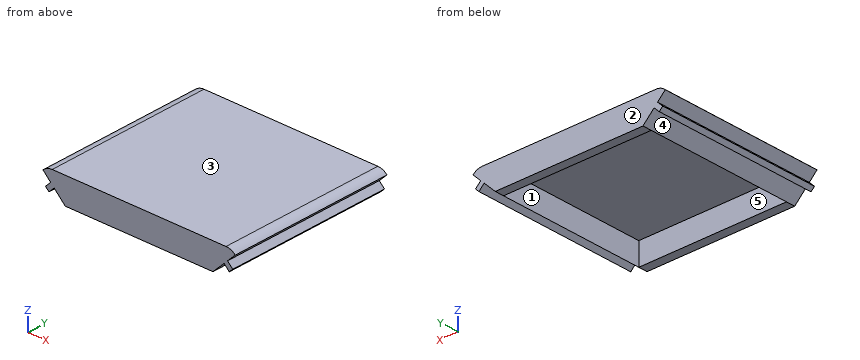
```python
from build123d import *

# Parameters (mm, degrees)
SKETCH_1_W          = 81.9
SKETCH_1_H          = 67.9
EXTRUDE_1_DEPTH     = 10.7
SKETCH_2_W          = 60.5
SKETCH_2_H          = 60.5
CUT_EXTRUDE_1_DEPTH = 9.2
CUT_EXTRUDE_2_REACH = 82.011
CUT_EXTRUDE_4_REACH = 91.242
EXTRUDE_2_DEPTH     = 67.9


with BuildPart() as part:
    # Эскиз1 → Бобышка-Вытянуть1 (new body)
    with BuildSketch(Plane.XY):
        Rectangle(SKETCH_1_W, SKETCH_1_H)
    extrude(amount=-EXTRUDE_1_DEPTH)

    # Эскиз2 → Вырез-Вытянуть1 (cut)
    with BuildSketch(Plane(origin=(0, 0, -10.7), x_dir=(-1, 0, 0), z_dir=(0, 0, -1))):
        Rectangle(SKETCH_2_W, SKETCH_2_H)
    extrude(amount=-CUT_EXTRUDE_1_DEPTH, mode=Mode.SUBTRACT)

    # Эскиз3 → Вырез-Вытянуть2 (cut, up to next)
    with BuildSketch(Plane(origin=(0, 33.95, 0), x_dir=(1, 0, 0), z_dir=(0, 1, 0)), mode=Mode.PRIVATE) as cut_extrude_2_sk1:
        Polygon((-40.95, 0), (-30.25, 10.7), (-40.95, 10.7), align=None)
    cut_extrude_2_tool1 = extrude(cut_extrude_2_sk1.sketch, amount=-CUT_EXTRUDE_2_REACH, mode=Mode.PRIVATE) & part.part
    # Эскиз3 → Вырез-Вытянуть2 (cut, up to next)
    with BuildSketch(Plane(origin=(0, 33.95, 0), x_dir=(1, 0, 0), z_dir=(0, 1, 0)), mode=Mode.PRIVATE) as cut_extrude_2_sk2:
        Polygon((40.95, 10.7), (40.95, 0), (30.25, 10.7), align=None)
    cut_extrude_2_tool2 = extrude(cut_extrude_2_sk2.sketch, amount=-CUT_EXTRUDE_2_REACH, mode=Mode.PRIVATE) & part.part
    add(cut_extrude_2_tool1.solids().sort_by_distance((-37.383333, 33.95, -7.133333))[0], mode=Mode.SUBTRACT)
    add(cut_extrude_2_tool2.solids().sort_by_distance((37.383333, 33.95, -7.133333))[0], mode=Mode.SUBTRACT)

    # Эскиз4 → Вырез-Вытянуть4 (cut, up to next)
    with BuildSketch(Plane(origin=(0, -33.95, -40.95), x_dir=(1, 0, 0), z_dir=(0, 1, 0)), mode=Mode.PRIVATE) as cut_extrude_4_sk1:
        with BuildLine():
            Line((39.383021279, -39.383021279), (40.95, -40.95))
            Line((40.95, -40.95), (35.6, -40.95))
            ThreePointArc((35.6, -40.95), (37.647356363, -40.542755499), (39.383021279, -39.383021279))
        make_face()
    cut_extrude_4_tool1 = extrude(cut_extrude_4_sk1.sketch, amount=CUT_EXTRUDE_4_REACH, mode=Mode.PRIVATE) & part.part
    # Эскиз4 → Вырез-Вытянуть4 (cut, up to next)
    with BuildSketch(Plane(origin=(0, -33.95, -40.95), x_dir=(1, 0, 0), z_dir=(0, 1, 0)), mode=Mode.PRIVATE) as cut_extrude_4_sk2:
        with BuildLine():
            Line((-40.95, -40.95), (-35.6, -40.95))
            ThreePointArc((-35.6, -40.95), (-37.647356363, -40.542755499), (-39.383021279, -39.383021279))
            Line((-39.383021279, -39.383021279), (-40.95, -40.95))
        make_face()
    cut_extrude_4_tool2 = extrude(cut_extrude_4_sk2.sketch, amount=CUT_EXTRUDE_4_REACH, mode=Mode.PRIVATE) & part.part
    add(cut_extrude_4_tool1.solids().sort_by_distance((39.042099, -33.95, -0.482136))[0], mode=Mode.SUBTRACT)
    add(cut_extrude_4_tool2.solids().sort_by_distance((-39.042099, -33.95, -0.482136))[0], mode=Mode.SUBTRACT)

    # Эскиз7 → Бобышка-Вытянуть2 (add)
    with BuildSketch(Plane(origin=(0, 33.95, 0), x_dir=(1, 0, 0), z_dir=(0, 1, 0))):
        Polygon((-38.352044546, 6.840596142), (-36.937830983, 8.254809704), (-34.81651064, 6.13348936), (-36.230724202, 4.719275798), align=None)
        Polygon((36.937830983, 8.254809704), (34.81651064, 6.13348936), (36.230724202, 4.719275798), (38.352044546, 6.840596142), align=None)
    extrude(amount=-EXTRUDE_2_DEPTH)


solid = part.part
```
Build history of the part. All positions in model axes, mm. Face numbers are marked on the shaded views. A direction names the side the tool comes from. Give positions to 0.01 mm unless a question says otherwise; leave off trailing zeros. Loops run counter-clockwise (first coordinate to the right, second up) from the corner with the lowest first, then second, coordinate; pieces in that order, holes last.
Item 1: Which spindle directions (+Z, -Z, +X, -X, +Y, -Y) get a long thin tool onto all of the face, cutting with end or side? Do the marked faces 3, 4 and 5. Say none if no direction does.
Answers follow:
face 3: +Z, +X, -X, +Y, -Y
face 4: -Z, +Y, -Y
face 5: -Z
Item 2: Drill centre lines: line 1 (X direction, y = -3, z = -4); line 2 (Y direction, x = -12, z = -4.75); line 3 (Z direction, x = -5, y = -20.5). Where is each one in solid material? Low to high.
Answers follow:
line 1: x = -36.95 to -30.25, 30.25 to 36.95
line 2: y = -33.95 to -30.25, 30.25 to 33.95
line 3: z = -1.5 to 0
Item 3: Flat gauge pins, fed straight in: pin 1 (4.5 mm diameter, centred on y = -10.5, z = -4.5, fed in from -X); pin 2 (6 mm diameter, centred on y = -11, z = -3, fed in from -X); pin 3 (3 mm diameter, centred on y = 26, z = -9.5, fed in from -X). Where does each tip first touch, or does it go through?
Answers follow:
pin 1: stops at x = -38.7
pin 2: stops at x = -39.38
pin 3: stops at x = -37.19
Item 4: Slice it at A-A, the plane z = -3.75. List the corners of the cut face in (x, y), and give its area (3 significant figures).
Answers follow:
outline: (-37.2, -33.95) - (37.2, -33.95) - (37.2, 33.95) - (-37.2, 33.95) - close; hole (-30.25, -30.25) - (30.25, -30.25) - (30.25, 30.25) - (-30.25, 30.25) - close
area: 1,390 mm2
Item 5: Slice it at C-C, the plane x = -14. List the corners of the cut face in (y, z).
Answers follow:
outline: (-33.95, -10.7) - (-30.25, -10.7) - (-30.25, -1.5) - (30.25, -1.5) - (30.25, -10.7) - (33.95, -10.7) - (33.95, 0) - (-33.95, 0) - close
Item 6: Pull direction X, two halves, no side cores. Call the marked faces 1 and 2: released by +X, released by -X, zero draft, split by the parting line, or undercut.
Answers follow:
face 1: undercut
face 2: zero draft
Item 7: Slice it at B-B, the plane y = 13.5. List the corners of the cut face in (x, z).
Answers follow:
outline: (-39.38, -1.57) - (-36.23, -4.72) - (-38.35, -6.84) - (-36.94, -8.25) - (-34.82, -6.13) - (-30.25, -10.7) - (-30.25, -1.5) - (30.25, -1.5) - (30.25, -10.7) - (34.82, -6.13) - (36.94, -8.25) - (38.35, -6.84) - (36.23, -4.72) - (39.38, -1.57) arc R5.35 ccw to (35.6, 0) - (-35.6, 0) arc R5.35 ccw to start
